Can you work these out from the model? Positions are in its coordinate system, mm. A direction names the side the tool comes from. Give positions to 0.01 mm unless a question says otherwise; leave off trailing zeros. Write each loop counter-clockwise with the first axis right and the second up, starting at its lowest first coordinate (ties: lowest second). Pieces come first, ordered by that corner, then holes. Notation, with made-up numbers: M 32.25,1 L 77.25,1 A21 ccw 77.25,23 Z; hole C 82.25,87.5 d8. An arc over 180 degrees is marked long. Use CSV: the item, a comma, the result in double quotes. Start each with the question number.
from build123d import *

# Parameters (mm, degrees)
F1_DEPTH = 63.5
F2_DEPTH = 25.4
F3_DEPTH = 7.9375
F5_R     = 6.35


with BuildPart() as f1:
    # F0 (on Front) → F1 (new body, symmetric)
    with BuildSketch(Plane.XZ):
        Polygon((22.225, 9.525), (-41.275, 9.525), (-41.275, -9.525), (41.275, -9.525), (41.275, 9.525), align=None)
    extrude(amount=F1_DEPTH, both=True)

    # F0 (on Front) → F2 (join, symmetric)
    with BuildSketch(Plane.XZ):
        with BuildLine():
            Line((22.225, 27.0002), (22.225, 9.525))
            Line((22.225, 9.525), (41.275, 9.525))
            Line((41.275, 9.525), (41.275, 27.0002))
            ThreePointArc((41.275, 27.0002), (45.92468, 38.22552), (57.15, 42.8752))
            Line((57.15, 42.8752), (60.325, 42.8752))
            Line((60.325, 42.8752), (60.325, 61.9252))
            Line((60.325, 61.9252), (57.15, 61.9252))
            add(Edge.make_bspline(
                [(53.120623, 61.691982), (54.477951, 61.800732), (55.821866, 61.878972), (57.15, 61.9252)],
                knots=[107.944302, 107.944302, 107.944302, 107.944302, 111.504536, 111.504536, 111.504536, 111.504536], degree=3))
            ThreePointArc((53.120623, 61.691982), (31.068574, 50.227658), (22.225, 27.0002))
        make_face()
    extrude(amount=F2_DEPTH, both=True)

    # F0 (on Front) → F3 (join, symmetric)
    with BuildSketch(Plane.XZ):
        with BuildLine():
            add(Edge.make_bspline(
                [(-41.275, 9.525), (-41.51543, 27.050941), (11.967215, 58.394754), (53.120623, 61.691982)],
                knots=[0, 0, 0, 0, 107.944302, 107.944302, 107.944302, 107.944302], degree=3))
            Line((-41.275, 9.525), (22.225, 9.525))
            Line((22.225, 9.525), (22.225, 27.0002))
            ThreePointArc((22.225, 27.0002), (31.068574, 50.227658), (53.120623, 61.691982))
        make_face()
    extrude(amount=F3_DEPTH, both=True)

    # F0 (on Front) → F4 (revolve)
    with BuildSketch(Plane.XZ):
        Polygon((60.325, 66.675), (60.325, 61.9252), (65.104299, 61.9252), (85.725, 61.9252), (85.725, 66.675), align=None)
        Polygon((65.104299, 61.9252), (60.325, 61.9252), (60.325, 42.8752), (65.104299, 42.8752), (85.725, 42.8752), (85.725, 61.9252), align=None)
        Polygon((65.104299, 42.8752), (60.325, 42.8752), (60.325, 38.1), (85.725, 38.1), (85.725, 42.8752), align=None)
    revolve(axis=Axis((60.325, 0, 52.3875), (0, 0, -1)))

    # F5
    f5_edges = [f1.edges().sort_by_distance(p)[0] for p in [
        (41.275, -63.5, 0),
        (-41.275, -63.5, 0),
        (41.275, 63.5, 0),
        (-41.275, 63.5, 0),
    ]]
    fillet(f5_edges, radius=F5_R)


solid = f1.part
(1) Will these pins go through, and if not, where does the flat tip stop? pin 1 Ø10 at (x, z) = (72.5, 46.5) entering from +Y; pin 2 Ø19 at (x, z) = (48, 35) entering from -Y; pin 3 Ø11 at (y, z) = (4, 0) entering from +X (3 decimals).
(2) Please list where these lines run through material, in increasing order: L1, parallel to X at y = -55, z = -3 (3 decimals); L2, parallel to Z at x = -17, y = -23.5 (3 decimals); L3, parallel to Y at x = 25.5, z = 38. Write a range as [from, to].
(3) I want a section at C-C (y = -37.5). Write out the boundary of the cut face in (x, z) (3 decimals).
(4) I want a section at B-B (x = 39). Write out the boundary of the cut face in (y, z) (3 decimals).
(5) Which directions (+Z, -Z, +X, -X, +Y, -Y) give clear straight access to the entire face, cutting with the end or side of a thin tool? Please do faces 1 (the face through (41.275, -1, 4)), 2 (the face through (37, -25.4, 36)), 3 (the face through (-2, -7.938, 29)).
Geometry results:
1,pin 1,"stops at y = 24.37"
1,pin 2,"stops at y = -25.4"
1,pin 3,"stops at x = 41.275"
2,L1,"x = [-41.275, 41.275]"
2,L2,"z = [-9.525, 9.525]"
2,L3,"y = [-25.4, 25.4]"
3,outline,"M -41.275,-9.525 L 41.275,-9.525 L 41.275,9.525 L -41.275,9.525 Z"
4,outline,"M -62.02,-9.525 L 62.02,-9.525 L 62.02,9.525 L 25.4,9.525 L 25.4,56.839 L 13.799,56.839 L 13.799,66.675 L -13.799,66.675 L -13.799,56.839 L -25.4,56.839 L -25.4,9.525 L -62.02,9.525 Z"
5,face 1,"-Z, +X, +Y, -Y"
5,face 2,"+Z, +X, -X, -Y"
5,face 3,"+Z, -X, -Y"
